The figure shows three views and two pictorial views of one solid part (mm, origin at its lowest corner). Answer the questions. Round coordinates to 2 decimals unless told otherwise and drop trailing zeros. Order: outer loops, then holes, each group sorted by start corner. A loop starts at its lowest first (then second) coordinate and runs counter-clockwise, first axis right, second up.
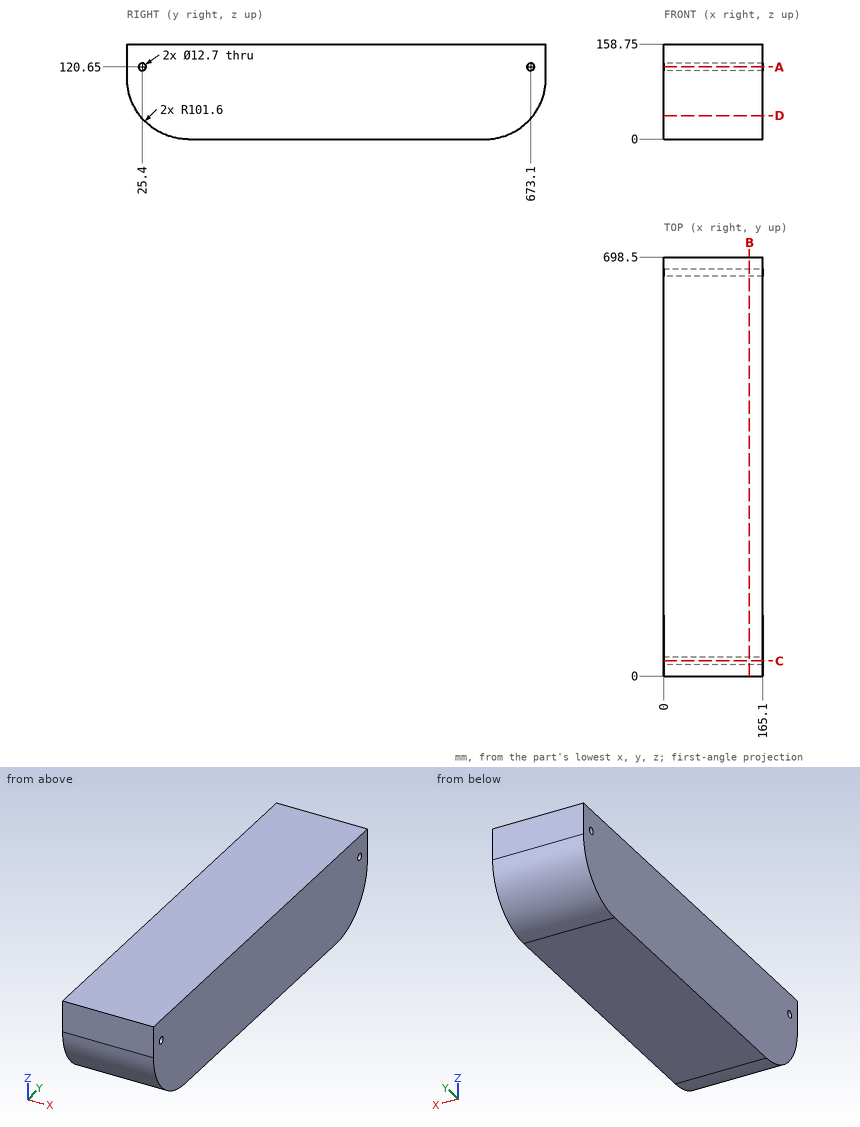
Item 1: Find section A-A (z = 120.65). Write down the section's boundary in (x, y).
Item 2: Given pin 1 (3 mm diameter, centred on x = 127.5, y = 261, fed in from -Z); pin 2 (11.5 mm diameter, centred on y = 673.1, z = 120.65, fed in from +X); pin 3 (1.5 mm diameter, centred on x = 59.5, z = 83.5, fed in from +Y); pin 4 (4 mm diameter, centred on x = 21, z = 26.5, fed in from +Y), each flat-ended and moving along its own axis, determine where each tip first touches the part or whether it passes through.
Item 3: Find section C-C (y = 25.4). Write down the section's boundary in (x, z), plus the area to 3 significant figures.
Item 4: Find section D-D (z = 39.5). Write down the section's boundary in (x, y).
Item 5: Find section B-B (x = 142.5). Write down the section's boundary in (y, z).
Item 6: Find the intervals of material crossed by line 1 along Y through (x, z) = (87, 120); line 2 along Y through (x, z) = (15.5, 116); line 3 along Z through (x, y) = (61, 673.1), in increasing order.
Model answer:
1. outline: (0, 0) - (165.1, 0) - (165.1, 19.05) - (0, 19.05) - close; (0, 31.75) - (165.1, 31.75) - (165.1, 666.75) - (0, 666.75) - close; (0, 679.45) - (165.1, 679.45) - (165.1, 698.5) - (0, 698.5) - close
2. pin 1: stops at z = 0
2. pin 2: passes through
2. pin 3: stops at y = 697.01
2. pin 4: stops at y = 667.46
3. outline: (0, 34.4) - (165.1, 34.4) - (165.1, 114.3) - (0, 114.3) - close; (0, 127) - (165.1, 127) - (165.1, 158.75) - (0, 158.75) - close
3. area: 18,400 mm2
4. outline: (0, 21.19) - (165.1, 21.19) - (165.1, 677.31) - (0, 677.31) - close
5. outline: (0, 101.6) arc R101.6 ccw to (101.6, 0) - (596.9, 0) arc R101.6 ccw to (698.5, 101.6) - (698.5, 158.75) - (0, 158.75) - close; hole circle Ø12.7 at (25.4, 120.65); hole circle Ø12.7 at (673.1, 120.65)
6. line 1: y = 0 to 19.08, 31.72 to 666.78, 679.42 to 698.5
6. line 2: y = 0 to 21.08, 29.72 to 668.78, 677.42 to 698.5
6. line 3: z = 34.4 to 114.3, 127 to 158.75
